Read the model definition and answer for the solid it produces. Units are mm, in the model's axes. Face numbers are marked on the shaded views. A direction names the side the tool comes from. Coordinates: 2 decimals unless noted, no trailing zeros. Loops run counter-clockwise (first coordinate to the right, second up) from the corner with the lowest first, then second, coordinate; pieces in that order, holes last.
Q1. Section C-C (z = -20) is taken. Give the vertices of the cut face in (x, y).
Q2. Flat-ended cylindrical pins translate along their axes: P1, Ø3, axis at x = -3.5, z = -31, coming from the +Y side; P2, Ø4, axis at x = 6.5, z = -14.5, coming from the +Y side. Find the tip coordinate at first contact, or state that the pin passes through.
Q3. Which of the six approach directions +Z, -Z, +X, -X, +Y, -Y give full straight-line access (tool end or side, diameter ignored) to the marked faces 1 and 2?
Q4. Straight lines are drawn through the part: line 1 (Z direction, x = 13, y = 23.5); line 2 (Z direction, x = -21, y = -18.5); line 3 (Y direction, x = -3, z = -26). For each, find the intervals that lie inside material, in ascending order.
from build123d import *

# Parameters (mm, degrees)
F0_R     = 30
F1_DEPTH = 5
F2_R     = 3
F3_R     = 1.99999
F4_R     = 5
F5_DEPTH = 82


# Not quite as in the source:
# - a fillet or chamfer is up to 0.001 mm smaller than in the source, because OpenCascade refuses the exact size


with BuildPart() as f1:
    # F0 (on Top) → F1 (new body)
    with BuildSketch(Plane.XY):
        Circle(F0_R)
    extrude(amount=F1_DEPTH)

    # F2
    f2_edges = [f1.edges().sort_by_distance(p)[0] for p in [
        (-30, 0, 5),
    ]]
    fillet(f2_edges, radius=F2_R)

    # F3 (radius 2 in the source; OpenCascade refuses exactly that, so slightly less here)
    f3_edges = [f1.edges().sort_by_distance(p)[0] for p in [
        (-30, 0, 0),
    ]]
    fillet(f3_edges, radius=F3_R)

    # F4 (on face) → F5 (join)
    with BuildSketch(Plane(origin=(0, 0, 0), x_dir=(1, 0, 0), z_dir=(0, 0, -1))):
        Circle(F4_R)
    extrude(amount=F5_DEPTH)


solid = f1.part
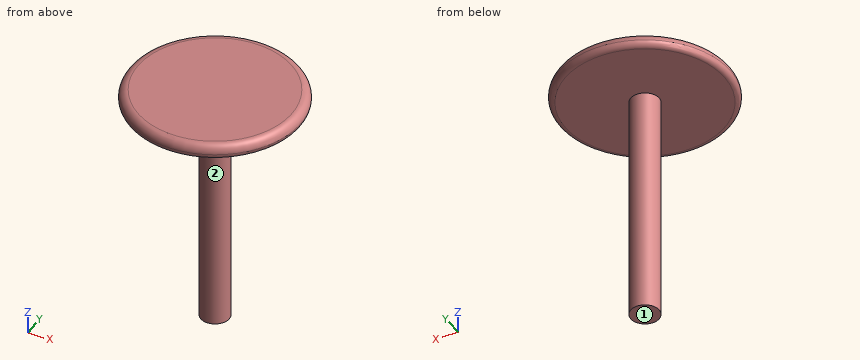
Numbers:
1. outline: circle Ø10 at (0, 0)
2. P1: stops at y = 4.58
2. P2: stops at y = 2.18
3. face 1: -Z, +X, -X, +Y, -Y
3. face 2: -Z
4. line 1: z = 0 to 5
4. line 2: z = 0 to 4.83
4. line 3: y = -4 to 4
